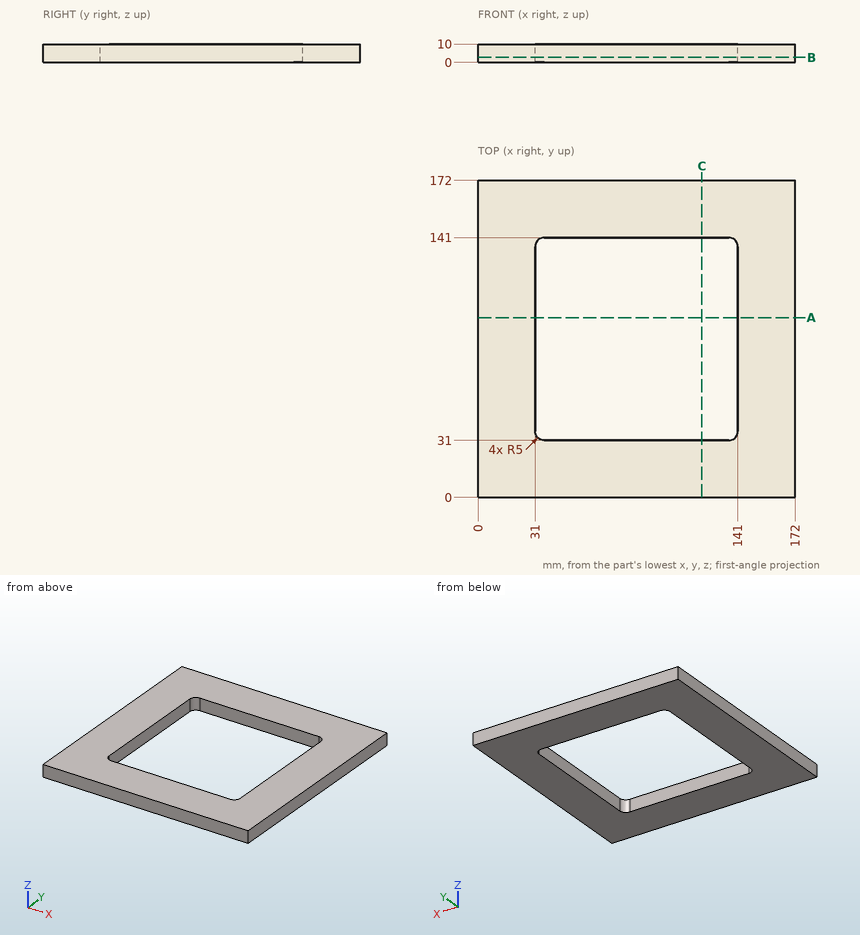
Verification items for this drawing (mm, ordinates from the low corner). Give positions to 0.01 mm unless a question says otherwise; leave off trailing zeros. Order: outer loops, then holes, each group sorted by start corner. A loop starts at its lowest first (then second) coordinate and runs counter-clockwise, first axis right, second up. Notation, with made-up numbers: M -2,45 L 36,45 A30 cw 36,78 Z; hole C 48.25,35.25 d8. An arc over 180 degrees is marked long. Use a Markdown table: item, result.
Item 1: Depth check by flat-ended pin: P1, Ø2, axis at y = 86.5, z = 1.5, coming from the -X side. Enter the tip coordinate at first touch or a pass-through.
Answers follow:
| item | result |
|---|---|
| P1 | stops at x = 0 |
Item 2: Material ranges on line 1 along X through (y, z) = (63, 6), recorded low to high.
Answers follow:
| item | result |
|---|---|
| line 1 | x = 0 to 31, 141 to 172 |
Item 3: Section check B-B (z = 2.75). Record the cut outline in (x, y), and give its area (3 significant figures).
Answers follow:
| item | result |
|---|---|
| outline | M 0,0 L 172,0 L 172,172 L 0,172 Z; hole M 31,36 A5 ccw 36,31 L 136,31 A5 ccw 141,36 L 141,136 A5 ccw 136,141 L 36,141 A5 ccw 31,136 Z |
| area | 17,500 mm2 |
Item 4: Section check A-A (y = 97.5). Record the cut outline in (x, z).
Answers follow:
| item | result |
|---|---|
| outline | M 0,0 L 31,0 L 31,10 L 0,10 Z; M 141,0 L 172,0 L 172,10 L 141,10 Z |
